Build history of the part. All positions in model axes, mm. A direction names the side the tool comes from. Round coordinates to 2 decimals unless told otherwise and drop trailing zeros. Write each loop counter-clockwise with the first axis right and the second up, starting at its lowest first coordinate (ties: lowest second). Pieces come first, ordered by that corner, then holes. Notation, with made-up numbers: (-17, 35.25) - (-13, 35.25) arc R28 ccw to (-13, 72.25) - close; hole circle Ø1 at (-33, 72.25). An arc over 180 degrees is marked (long way). One line per question, with ' | ' between items.
from build123d import *

# Parameters (mm, degrees)
SKIZZE1_W                       = 20.1
SKIZZE1_H                       = 13
AUFSATZ_LINEAR_AUSTRAGEN1_DEPTH = 11
SKIZZE2_W                       = 0.5
SKIZZE2_H                       = 5
AUFSATZ_LINEAR_AUSTRAGEN2_DEPTH = 8.7
SKIZZE4_R                       = 0.706106742
SCHNITT_LINEAR_AUSTRAGEN1_DEPTH = 8.7
FASE1_SIZE                      = 1
SKIZZE5_W                       = 23.1
SKIZZE5_H                       = 16
AUFSATZ_LINEAR_AUSTRAGEN3_DEPTH = 2
AUFSATZ_LINEAR_AUSTRAGEN4_DEPTH = 13


with BuildPart() as part:
    # Skizze1 → Aufsatz-Linear austragen1 (new body)
    with BuildSketch(Plane.XY):
        with Locations((10.05, -6.5)):
            Rectangle(SKIZZE1_W, SKIZZE1_H)
    extrude(amount=AUFSATZ_LINEAR_AUSTRAGEN1_DEPTH)

    # Skizze2 → Aufsatz-Linear austragen2 (add)
    with BuildSketch(Plane.XY.offset(11)):
        with Locations((2.25, -6.5)):
            Rectangle(SKIZZE2_W, SKIZZE2_H)
        with Locations((9.35, -6.5)):
            Rectangle(SKIZZE2_W, SKIZZE2_H)
    extrude(amount=AUFSATZ_LINEAR_AUSTRAGEN2_DEPTH)

    # Skizze4 → Schnitt-Linear austragen1 (cut)
    with BuildSketch(Plane.ZY.offset(-2)):
        with Locations((17.612214696, -6.5)):
            Circle(SKIZZE4_R)
    extrude(amount=-SCHNITT_LINEAR_AUSTRAGEN1_DEPTH, mode=Mode.SUBTRACT)

    # Fase1
    fase1_edges = [part.edges().sort_by_distance(p)[0] for p in [
        (2.25, -4, 19.7),
        (2.25, -9, 19.7),
        (9.35, -9, 19.7),
        (9.35, -4, 19.7),
    ]]
    chamfer(fase1_edges, length=FASE1_SIZE)

    # Skizze5 → Aufsatz-Linear austragen3 (add)
    with BuildSketch(Plane(origin=(0, 0, 0), x_dir=(-1, 0, 0), z_dir=(0, 0, -1))):
        with Locations((-10.05, -6.5)):
            Rectangle(SKIZZE5_W, SKIZZE5_H)
    extrude(amount=AUFSATZ_LINEAR_AUSTRAGEN3_DEPTH)

    # Skizze6 → Aufsatz-Linear austragen4 (add)
    with BuildSketch(Plane(origin=(0, 0, 0), x_dir=(1, 0, 0), z_dir=(0, 1, 0))):
        with BuildLine():
            Line((0, 2), (1.361035654, 8.016649053))
            ThreePointArc((1.361035654, 8.016649053), (10.576058723, 4.527258802), (20.1, 2))
            Line((20.1, 2), (0, 2))
        make_face()
    extrude(amount=-AUFSATZ_LINEAR_AUSTRAGEN4_DEPTH)


solid = part.part
Q1. Which spindle directions (+Z, -Z, +X, -X, +Y, -Y) get a long thin tool onto all of the face, cutting with end or side? Do faces 1 (the flat face through (10.2, -13.5, -2)), 2 (the flat face through (6, 0, -4)), 3 (the flat face through (10, 0, 5)), 4 (the flat face through (6, -13, -4)). Say none if no direction does.
Found:
face 1: -Z | face 2: -Z, +X, -X, +Y | face 3: +Z, +X, -X, +Y | face 4: -Z, +X, -X, -Y
Q2. Drop flat-ended pins along their axis: pin 1 (6 mm diameter, centred on x = 6, y = -8.5, fed in from +Z); pin 2 (1 mm diameter, centred on y = -1, z = 8.5, fed in from +X); pin 3 (1.5 mm diameter, centred on y = -7.5, z = 17.5, fed in from +X). Give the stop position or say it passes through.
Found:
pin 1: z = 11 | pin 2: x = 20.1 | pin 3: x = 9.6
Q3. Drill centre lines: L1, parallel to Y at x = 18.75, z = 8.75; L2, parallel to Z at x = 7.75, y = -13.5; L3, parallel to X at y = -5, z = 3. Where is each one in solid material? Low to high. Write a range as from..to.
Found:
L1: -13..0 | L2: -2..0 | L3: 0..20.1
Q4. Saw through at A-A, the plane y = -6.5. List the corners of the cut face in (x, z).
Found:
outline: (-1.5, -2) - (0, -2) - (1.36, -8.02) arc R96.08 cw to (20.1, -2) - (21.6, -2) - (21.6, 0) - (20.1, 0) - (20.1, 11) - (9.6, 11) - (9.6, 16.91) - (9.1, 16.91) - (9.1, 11) - (2.5, 11) - (2.5, 16.91) - (2, 16.91) - (2, 11) - (0, 11) - (0, 0) - (-1.5, 0) - close; (2, 18.32) - (2.5, 18.32) - (2.5, 19.7) - (2, 19.7) - close; (9.1, 18.32) - (9.6, 18.32) - (9.6, 19.7) - (9.1, 19.7) - close
Q5. Saw through at C-C, the plane y = -3.25. List the corners of the cut face in (x, z).
Found:
outline: (-1.5, -2) - (0, -2) - (1.36, -8.02) arc R96.08 cw to (20.1, -2) - (21.6, -2) - (21.6, 0) - (20.1, 0) - (20.1, 11) - (0, 11) - (0, 0) - (-1.5, 0) - close
Q6. Pull direction X, two halves, no side cores. Call faces 5 (the flat face through (9.1, -7, 15)), 6 (the cylindrical face through (10.44, -6.41, -4.57)), 7 (the flat face through (10.2, -13.5, 0)): +X half, -X half, draft (parallel to the pull), parting line (faces both ways), or undercut.
Found:
face 5: undercut | face 6: +X half | face 7: draft
Q7. Saw through at B-B, the plane z = 15. List the corners of the cut face in (x, y).
Found:
outline: (2, -9) - (2.5, -9) - (2.5, -4) - (2, -4) - close; (9.1, -9) - (9.6, -9) - (9.6, -4) - (9.1, -4) - close
Q8. Saw through at D-D, the plane x = 18.25. List the corners of the cut face in (y, z), then the cut area to 3 significant figures.
Found:
outline: (-14.5, -2) - (-13, -2) - (-13, -2.41) - (0, -2.41) - (0, -2) - (1.5, -2) - (1.5, 0) - (0, 0) - (0, 11) - (-13, 11) - (-13, 0) - (-14.5, 0) - close | area: 180 mm^2
